from build123d import *

# Parameters (mm, degrees)
F0_W     = 128
F0_H     = 86.5
F0_W_2   = 93.25
F0_H_2   = 54.5
F1_DEPTH = 2
F2_W     = 3.2
F2_H     = 82.5
F2_H_2   = 2
F2_W_2   = 121.6
F3_DEPTH = 8
F4_R     = 1


with BuildPart() as f1:
    # F0 (on Top) → F1 (new body)
    with BuildSketch(Plane.XY):
        Rectangle(F0_W, F0_H)
        Rectangle(F0_W_2, F0_H_2, mode=Mode.SUBTRACT)
    extrude(amount=F1_DEPTH)

    # F2 (on face) → F3 (join)
    with BuildSketch(Plane.XY.offset(2)):
        with Locations((-62.4, 0)):
            Rectangle(F2_W, F2_H)
        with Locations((-62.4, 42.25)):
            Rectangle(F2_W, F2_H_2)
        with Locations((0, 42.25)):
            Rectangle(F2_W_2, F2_H_2)
        with Locations((62.4, 42.25)):
            Rectangle(F2_W, F2_H_2)
        with Locations((62.4, 0)):
            Rectangle(F2_W, F2_H)
        with Locations((62.4, -42.25)):
            Rectangle(F2_W, F2_H_2)
        with Locations((0, -42.25)):
            Rectangle(F2_W_2, F2_H_2)
        with Locations((-62.4, -42.25)):
            Rectangle(F2_W, F2_H_2)
    extrude(amount=F3_DEPTH)

    # F4
    f4_edges = [f1.edges().sort_by_distance(p)[0] for p in [
        (-64, -43.25, 5),
        (-64, 43.25, 5),
        (64, -43.25, 5),
        (64, 43.25, 5),
    ]]
    fillet(f4_edges, radius=F4_R)


solid = f1.part
Input: part model. Units: mm. Frame: model coordinates. A direction names the side the tool comes from. Coordinates: 2 decimals unless noted, no trailing zeros. Loops run counter-clockwise (first coordinate to the right, second up) from the corner with the lowest first, then second, coordinate; pieces in that order, holes last. Notation, with made-up numbers: (31.25, 33) -> (85.25, 33) arc R31 ccw to (85.25, 67) -> close; hole circle Ø3 at (18, 42.25). An arc over 180 degrees is marked (long way). Write item = value, one per line. Start each with the question number.
Item 1: Reachability of faces 4 (the face through (-1, 28, 2)), 5 (the face through (1, 43.25, 5)) from +Z, -Z, +X, -X, +Y, -Y: full face, straight path, thin tool, end or side. Return the list, or none.
Item 2: Cut plane A-A, the plane y = -22. Return loops of the section in (x, z) (3 decimals).
Item 3: Cut plane B-B, the plane x = -18. Return loops of the section in (y, z).
Item 4: Mould query, pull axis X, two halves, no side actions, for faces 1 (the face through (-1, 41.25, 6)), 2 (the face through (-1, 29, 0)), 3 (the face through (64, -1, 5)). Classes: pulls with the +X half, pulls with the -X half, needs draft (parallel to the pull), parting line crosses it, or undercut.
Item 5: Cut plane C-C, the plane z = 8. Return loops of the section in (x, y), plus the area to 3 significant figures.
Item 6: First-contact query: P1, Ø2, axis at x = 13.5, y = -28, coming from the +Z side. Flat tip, straight axial feed; report the tip coordinate or a pass-through.
Item 7: Material intervals for line 1 (X direction, y = 24, z = 7.25); line 2 (Y direction, x = 33, z = 5.5); line 3 (X direction, y = -17.5, z = 1.5) (3 decimals), sorted ascending.
Item 8: Cut plane D-D, the plane x = 51.5. Return loops of the section in (y, z), plus the area to 3 significant figures.
Ans:
q1.face_4 = +Z
q1.face_5 = +Z, -Z, +X, -X, +Y
q2.outline = (-64, 0) -> (-46.625, 0) -> (-46.625, 2) -> (-60.8, 2) -> (-60.8, 10) -> (-64, 10) -> close; (46.625, 0) -> (64, 0) -> (64, 10) -> (60.8, 10) -> (60.8, 2) -> (46.625, 2) -> close
q3.outline = (-43.25, 0) -> (-27.25, 0) -> (-27.25, 2) -> (-41.25, 2) -> (-41.25, 10) -> (-43.25, 10) -> close; (27.25, 0) -> (43.25, 0) -> (43.25, 10) -> (41.25, 10) -> (41.25, 2) -> (27.25, 2) -> close
q4.face_1 = undercut
q4.face_2 = needs draft
q4.face_3 = pulls with the +X half
q5.outline = (-64, -42.25) arc R1 ccw to (-63, -43.25) -> (63, -43.25) arc R1 ccw to (64, -42.25) -> (64, 42.25) arc R1 ccw to (63, 43.25) -> (-63, 43.25) arc R1 ccw to (-64, 42.25) -> close; hole (-60.8, -41.25) -> (60.8, -41.25) -> (60.8, 41.25) -> (-60.8, 41.25) -> close
q5.area = 1,040 mm²
q6.P1 = 2
q7.line_1 = -64 to -60.8, 60.8 to 64
q7.line_2 = -43.25 to -41.25, 41.25 to 43.25
q7.line_3 = -64 to -46.625, 46.625 to 64
q8.outline = (-43.25, 0) -> (43.25, 0) -> (43.25, 10) -> (41.25, 10) -> (41.25, 2) -> (-41.25, 2) -> (-41.25, 10) -> (-43.25, 10) -> close
q8.area = 205 mm²
